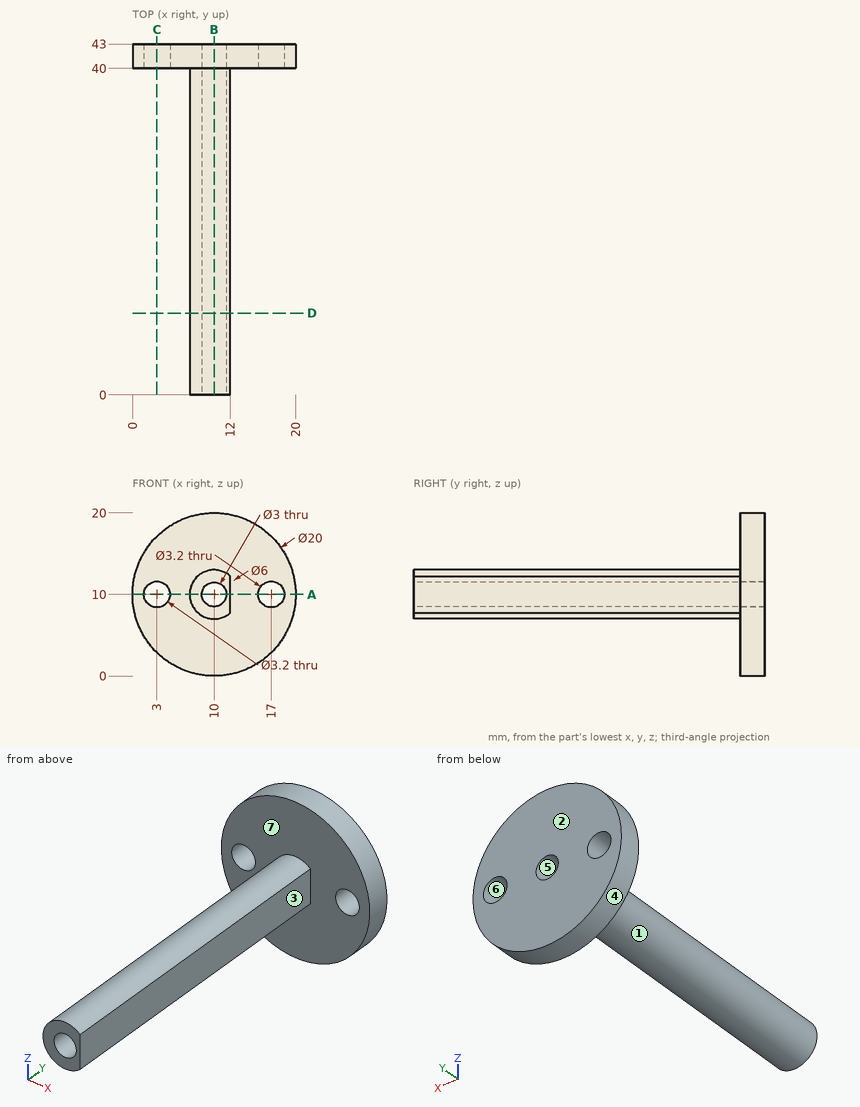
Drawing for the job (mm, zero at the part's lowest x, y, z). A direction names the side the tool comes from. Round coordinates to 2 decimals unless told otherwise and drop trailing zeros. Write each loop counter-clockwise with the first axis right and the second up, starting at its lowest first coordinate (ties: lowest second). Pieces come first, ordered by that corner, then holes. Notation, with made-up numbers: M 70,65 L 96,65 A19 ccw 96,88 Z; hole C 42,42.5 d3. An arc over 180 degrees is marked long. Put each result on its own line as item: value.
Item 1: Flat gauge pins, fed straight in: P1, Ø6, axis at x = 4, z = 6.5, coming from the -Y side; P2, Ø4, axis at x = 10, z = 10, coming from the -Y side; P3, Ø5, axis at y = 35, z = 16, coming from the +X side; P4, Ø6, axis at y = 26.5, z = 14, coming from the +X side. Where does each tip first touch, or does it go through?
Responses:
P1: y = 40
P2: y = 0
P3: through
P4: x = 12
Item 2: Cut at A-A (z = 10). List the corners of the cut face in (x, y).
Responses:
outline: M 0,40 L 1.4,40 L 1.4,43 L 0,43 Z; M 4.6,40 L 7,40 L 7,0 L 8.5,0 L 8.5,43 L 4.6,43 Z; M 11.5,0 L 12,0 L 12,40 L 15.4,40 L 15.4,43 L 11.5,43 Z; M 18.6,40 L 20,40 L 20,43 L 18.6,43 Z
Item 3: Probe L1, parallel to X at y = 40.95, z = 10; L2, parallel to X at y = 13, z = 10; L3, parallel to Y at x = 4, z = 4.75. List the from-to ranges inside material, lowest first. Write a range as from..to.
Responses:
L1: 0..1.4, 4.6..8.5, 11.5..15.4, 18.6..20
L2: 7..8.5, 11.5..12
L3: 40..43
Item 4: Cut at B-B (x = 10). List the corners of the cut face in (y, z), and give its area (3 significant figures).
Responses:
outline: M 0,7 L 40,7 L 40,0 L 43,0 L 43,8.5 L 0,8.5 Z; M 0,11.5 L 43,11.5 L 43,20 L 40,20 L 40,13 L 0,13 Z
area: 171 mm²
Item 5: Mould opens along X. For the marked faces 4, 5, 6 and 7 say: +X half, -X half, draft (parallel to the pull), parting line (faces both ways), or undercut.
Responses:
face 4: parting line
face 5: undercut
face 6: undercut
face 7: draft
Item 6: Cut at C-C (x = 3). List the corners of the cut face in (y, z), and give its area (3 significant figures).
Responses:
outline: M 40,2.86 L 43,2.86 L 43,8.4 L 40,8.4 Z; M 40,11.6 L 43,11.6 L 43,17.14 L 40,17.14 Z
area: 33.2 mm²
Item 7: Tool access for the marked faces 1, 2 and 3: list every direction of +Z, -Z, +X, -X, +Y, -Y with a clear straight run to the whole face (end or side of a thin tool).
Responses:
face 1: -Y
face 2: +Z, -Z, +X, -X, +Y
face 3: +Z, -Z, +X, -Y
Item 8: Cut at D-D (y = 10). List the corners of the cut face in (x, z), and give its area (3 significant figures).
Responses:
outline: M 12,7.76 L 12,12.24 A3 ccw long Z; hole C 10,10 d3
area: 18.1 mm²
